Design review of the part built by this model. Coordinates are the model's own, in mm. A direction names the side the tool comes from. Coordinates: 2 decimals unless noted, no trailing zeros. Loops run counter-clockwise (first coordinate to the right, second up) from the corner with the lowest first, then second, coordinate; pieces in that order, holes last. Notation, with made-up numbers: (-20, 68) - (0, 68) arc R8 cw to (0, 77) - close; hole circle Ø7 at (68.5, 60.5). An arc over 180 degrees is marked (long way). Use one line per item in the form item = value. Start each with the question number.
(1) Add section C-C (z = 4.45). State the section outline as (x, y) points.
(2) Tool access review of faces 5 (the face through (30, 6, 2)), 6 (the face through (30, 32, 2)): name each direction out of +Z, -Z, +X, -X, +Y, -Y from which nothing blocks a thin tool from reaching the whole face with its end or side.
(3) For L1, parallel to Y at x = 5.7, z = 2.9; L2, parallel to Y at x = 47, z = 0.95; L3, parallel to X at y = 14.5, z = 2.8, list the stretches that pass through material, from the lowest coordinate up.
(4) The part is to be moulded in two halves that separate along X. For faces 1 (the face through (6.6, 22.73, 2.46)), 2 (the face through (0, 16, 2)), 3 (the face through (60, 16, 2)), 4 (the face through (30, 0, 2)), say which applies: pulls with the +X half, pulls with the -X half, needs draft (parallel to the pull), parting line crosses it, or undercut.
(5) Add section B-B (x = 11). State the section outline as (y, z) points.
(6) Add section D-D (y = 23.5). State the section outline as (x, z) points.
(7) Add section A-A (y = 11). State the section outline as (x, z) points.
Autodesk Inventor part; units mm, degrees
ref_plane "YZ Plane" through (0, 0, 0) normal (1, 0, 0) x (0, 1, 0)
ref_plane "XZ Plane" through (0, 0, 0) normal (0, 1, 0) x (-1, 0, 0)
ref_plane "XY Plane" through (0, 0, 0) normal (0, 0, 1) x (1, 0, 0)
sketch "スケッチ2" plane through (0, 0, 0) normal (0, 0, 1) x (1, 0, 0)
  line L0 (0, 0) -> (60, 0)
  line L1 (60, 0) -> (60, 32)
  line L2 (60, 32) -> (0, 32)
  line L3 (0, 32) -> (0, 0)
  line L4 (3, 26) -> (57, 26)
  line L5 (57, 26) -> (57, 6)
  line L6 (57, 6) -> (3, 6)
  line L7 (3, 6) -> (3, 26)
  circle A0 centre (5.7, 21) radius 1.95
  circle A1 centre (5.7, 11) radius 1.95
  circle A2 centre (54.3, 21) radius 1.95
  circle A3 centre (54.3, 11) radius 1.95
  line L8 (9.55, 26) -> (50.45, 26)
  line L9 (50.45, 26) -> (50.45, 6)
  line L10 (50.45, 6) -> (9.55, 6)
  line L11 (9.55, 6) -> (9.55, 26)
  point P0 (30, 0)
  point P1 (9.55, 6)
  dimension "d78" = 20
  dimension "d79" = 3.9
  dimension "d80" = 3.9
  dimension "d81" = 3.9
  dimension "d82" = 3.9
  dimension "d83" = 48.6
  dimension "d84" = 54
  dimension "d85" = 2.7
  dimension "d86" = 2.7
  dimension "d87" = 48.6
  dimension "d88" = 10
  dimension "d89" = 5
  dimension "d90" = 10
  dimension "d91" = 5
  dimension "d92" = 60
  dimension "d93" = 3
  dimension "d94" = 40.9
  dimension "d95" = 6.55
  dimension "d96" = 6.55
  dimension "d97" = 32
  dimension "d98" = 6
extrude "押し出し2" add sketch "スケッチ2" along normal blind 5 contours L3 L2 L1 L0 | L4 L11 L6 L7 | L4 L5 L6 L9
equation "\"d80\" = d79"
equation "\"d81\" = d79"
equation "\"d82\" = d79"
equation "\"d86\" = d85"
equation "\"d87\" = d83"
equation "\"d90\" = d88"
equation "\"d91\" = d89"
properties part number "servo_case"
Computed values:
q1.outline = (0, 0) - (60, 0) - (60, 32) - (0, 32) - close; hole circle Ø3.9 at (5.7, 11); hole circle Ø3.9 at (5.7, 21); hole (9.55, 6) - (50.45, 6) - (50.45, 26) - (9.55, 26) - close; hole circle Ø3.9 at (54.3, 11); hole circle Ø3.9 at (54.3, 21)
q2.face_5 = +Z, -Z
q2.face_6 = +Z, -Z, +X, -X, +Y
q3.L1 = 0 to 9.05, 12.95 to 19.05, 22.95 to 32
q3.L2 = 0 to 6, 26 to 32
q3.L3 = 0 to 9.55, 50.45 to 60
q4.face_1 = undercut
q4.face_2 = pulls with the -X half
q4.face_3 = pulls with the +X half
q4.face_4 = needs draft
q5.outline = (0, 0) - (6, 0) - (6, 5) - (0, 5) - close; (26, 0) - (32, 0) - (32, 5) - (26, 5) - close
q6.outline = (0, 0) - (9.55, 0) - (9.55, 5) - (0, 5) - close; (50.45, 0) - (60, 0) - (60, 5) - (50.45, 5) - close
q7.outline = (0, 0) - (3.75, 0) - (3.75, 5) - (0, 5) - close; (7.65, 0) - (9.55, 0) - (9.55, 5) - (7.65, 5) - close; (50.45, 0) - (52.35, 0) - (52.35, 5) - (50.45, 5) - close; (56.25, 0) - (60, 0) - (60, 5) - (56.25, 5) - close
